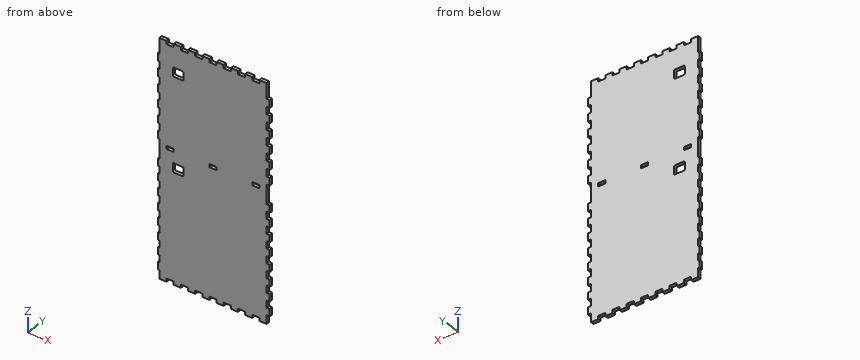
from build123d import *

# Parameters (mm, degrees)
F0_W     = 40
F0_H     = 18
F1_DEPTH = 18


with BuildPart() as f1:
    # F0 (on Front) → F1 (new body)
    with BuildSketch(Plane.XZ):
        Polygon((1349.999516, 1218), (1331.999516, 1218), (1331.999516, 1304), (1291.999516, 1304), (1291.999516, 1286), (1251.999516, 1286), (1251.999516, 1304), (1211.999516, 1304), (1211.999516, 1286), (1171.999516, 1286), (1171.999516, 1304), (1131.999516, 1304), (1131.999516, 1286), (1091.999516, 1286), (1091.999516, 1304), (1051.999516, 1304), (1051.999516, 1286), (1011.999516, 1286), (1011.999516, 1304), (971.999516, 1304), (971.999516, 1286), (931.999516, 1286), (931.999516, 1304), (891.999516, 1304), (891.999516, 1286), (851.999516, 1286), (851.999516, 1304), (811.999516, 1304), (811.999516, 1286), (771.999516, 1286), (771.999516, 1304), (731.999516, 1304), (731.999516, 1218), (722.999516, 1218), (722.999516, 1176), (731.999516, 1176), (731.999516, 1134), (722.999516, 1134), (722.999516, 1092), (731.999516, 1092), (731.999516, 1050), (722.999516, 1050), (722.999516, 1008), (731.999516, 1008), (731.999516, 966), (722.999516, 966), (722.999516, 924), (731.999516, 924), (731.999516, 882), (722.999516, 882), (722.999516, 840), (731.999516, 840), (731.999516, 798), (722.999516, 798), (722.999516, 756), (731.999516, 756), (731.999516, 648), (722.999516, 648), (722.999516, 608), (731.999516, 608), (731.999516, 568), (722.999516, 568), (722.999516, 528), (731.999516, 528), (731.999516, 488), (722.999516, 488), (722.999516, 448), (731.999516, 448), (731.999516, 408), (722.999516, 408), (722.999516, 368), (731.999516, 368), (731.999516, 328), (722.999516, 328), (722.999516, 288), (731.999516, 288), (731.999516, 248), (722.999516, 248), (722.999516, 208), (731.999516, 208), (731.999516, 168), (722.999516, 168), (722.999516, 128), (731.999516, 128), (731.999516, 88), (722.999516, 88), (722.999516, 48), (731.999516, 48), (731.999516, 0), (771.999516, 0), (771.999516, 18), (811.999516, 18), (811.999516, 0), (851.999516, 0), (851.999516, 18), (891.999516, 18), (891.999516, 0), (931.999516, 0), (931.999516, 18), (971.999516, 18), (971.999516, 0), (1011.999516, 0), (1011.999516, 18), (1051.999516, 18), (1051.999516, 0), (1091.999516, 0), (1091.999516, 18), (1131.999516, 18), (1131.999516, 0), (1171.999516, 0), (1171.999516, 18), (1211.999516, 18), (1211.999516, 0), (1251.999516, 0), (1251.999516, 18), (1291.999516, 18), (1291.999516, 0), (1331.999516, 0), (1331.999516, 48), (1349.999516, 48), (1349.999516, 88), (1331.999516, 88), (1331.999516, 128), (1349.999516, 128), (1349.999516, 168), (1331.999516, 168), (1331.999516, 208), (1349.999516, 208), (1349.999516, 248), (1331.999516, 248), (1331.999516, 288), (1349.999516, 288), (1349.999516, 328), (1331.999516, 328), (1331.999516, 368), (1349.999516, 368), (1349.999516, 408), (1331.999516, 408), (1331.999516, 448), (1349.999516, 448), (1349.999516, 488), (1331.999516, 488), (1331.999516, 528), (1349.999516, 528), (1349.999516, 568), (1331.999516, 568), (1331.999516, 608), (1349.999516, 608), (1349.999516, 648), (1331.999516, 648), (1331.999516, 756), (1349.999516, 756), (1349.999516, 798), (1331.999516, 798), (1331.999516, 840), (1349.999516, 840), (1349.999516, 882), (1331.999516, 882), (1331.999516, 924), (1349.999516, 924), (1349.999516, 966), (1331.999516, 966), (1331.999516, 1008), (1349.999516, 1008), (1349.999516, 1050), (1331.999516, 1050), (1331.999516, 1092), (1349.999516, 1092), (1349.999516, 1134), (1331.999516, 1134), (1331.999516, 1176), (1349.999516, 1176), align=None)
        with BuildLine():
            Line((806.999516, 614), (806.999516, 652))
            ThreePointArc((806.999516, 652), (808.756876, 656.242641), (812.999516, 658))
            Line((812.999516, 658), (860.999516, 658))
            ThreePointArc((860.999516, 658), (865.242157, 656.242641), (866.999516, 652))
            Line((866.999516, 652), (866.999516, 614))
            ThreePointArc((866.999516, 614), (865.242157, 609.757359), (860.999516, 608))
            Line((860.999516, 608), (812.999516, 608))
            ThreePointArc((812.999516, 608), (808.756876, 609.757359), (806.999516, 614))
        make_face(mode=Mode.SUBTRACT)
        with Locations((791.999516, 727)):
            Rectangle(F0_W, F0_H, mode=Mode.SUBTRACT)
        with Locations((1031.999516, 727)):
            Rectangle(F0_W, F0_H, mode=Mode.SUBTRACT)
        with BuildLine():
            ThreePointArc((860.999516, 1176), (865.242157, 1174.242641), (866.999516, 1170))
            Line((866.999516, 1170), (866.999516, 1132))
            ThreePointArc((866.999516, 1132), (865.242157, 1127.757359), (860.999516, 1126))
            Line((860.999516, 1126), (812.999516, 1126))
            ThreePointArc((812.999516, 1126), (808.756876, 1127.757359), (806.999516, 1132))
            Line((806.999516, 1132), (806.999516, 1170))
            ThreePointArc((806.999516, 1170), (808.756876, 1174.242641), (812.999516, 1176))
            Line((812.999516, 1176), (860.999516, 1176))
        make_face(mode=Mode.SUBTRACT)
        with Locations((1271.999516, 727)):
            Rectangle(F0_W, F0_H, mode=Mode.SUBTRACT)
    extrude(amount=F1_DEPTH)


solid = f1.part
Read the model definition and answer for the solid it produces. Units are mm, in the model's axes. Give positions to 0.01 mm unless a question says otherwise; leave off trailing zeros. Write each loop counter-clockwise with the first axis right and the second up, starting at its lowest first coordinate (ties: lowest second). Pieces come first, ordered by that corner, then holes. Notation, with made-up numbers: (52, 86) - (80, 86) arc R18 cw to (80, 111) - close; hole circle Ø3 at (32.25, 62.25). An arc over 180 degrees is marked (long way). Use CSV: the item, a comma, the result in double quotes. Start each with the question number.
Item 1: Consider line 1 (Z direction, x = 828.5, y = -17); line 2 (Z direction, x = 853, y = -3.25); line 3 (Z direction, x = 806.5, y = -1). Determine where each line is inside the solid, lowest interval first.
Item 2: The part is cut by section B-B, the plane y = -14.5. Count the separate pieces of the cut face and the enclosed holes in it, and give its area (3 significant figures).
Item 3: The part is cut by section C-C, the plane z = 263. Give the vertices of the cut face in (x, y), and give its area (3 significant figures).
Item 4: Flat-ended cylindrical pins translate along their axes: P1, Ø4, axis at x = 1272, y = -7, coming from the -Z side; P2, Ø9, axis at y = -11.5, z = 1072, coming from the +X side; P3, Ø4.5, axis at x = 725.5, y = -4.5, coming from the -Z side. Find the tip coordinate at first contact, or state that the pin passes through.
Item 5: The part is cut by section A-A, the plane x = 1111. Give the vertices of the cut face in (y, z).
Taken from the geometry:
1,line 1,"0 to 608, 658 to 1126, 1176 to 1304"
1,line 2,"18 to 608, 658 to 1126, 1176 to 1286"
1,line 3,"18 to 718, 736 to 1286"
2,separate pieces,"1"
2,enclosed holes,"5"
2,area,"780,000 mm2"
3,outline,"(732, -18) - (1332, -18) - (1332, 0) - (732, 0) - close"
3,area,"10,800 mm2"
4,P1,"z = 18"
4,P2,"x = 1332"
4,P3,"z = 48"
5,outline,"(-18, 18) - (0, 18) - (0, 1286) - (-18, 1286) - close"
